from build123d import *

# Parameters (mm, degrees)
SKETCH1_W           = 52
SKETCH1_H           = 38
BULK_EXTRUDE_DEPTH  = 3
FILLET1_R           = 7
SKETCH2_R           = 31.5
MOTOR_SUPPORT_DEPTH = 3
SKETCH3_R           = 6
WIRE_PASSTHRU_DEPTH = 143.168954603
FILLET2_R           = 10


with BuildPart() as part:
    # Sketch1 → BULK EXTRUDE (new body)
    # profile 1 of 3: a face of its own
    with BuildSketch(Plane.ZY.offset(19)):
        with BuildLine():
            Line((-2, -62.201941274), (-2, -24.5))
            Line((-2, -24.5), (-2, 25.456486729))
            ThreePointArc((-2, 25.456486729), (-115, -18.372727273), (-2, -62.201941274))
        make_face()
        with Locations((-57, 0)):
            Rectangle(SKETCH1_W, SKETCH1_H, mode=Mode.SUBTRACT)
    # profile 2 of 3: a face of its own
    with BuildSketch(Plane.ZY.offset(19)):
        with Locations((-57, 0)):
            Rectangle(SKETCH1_W, SKETCH1_H)
    # profile 3 of 3: a face of its own
    with BuildSketch(Plane.ZY.offset(19)):
        with BuildLine():
            Line((14.71055964, -24.5), (-2, -24.5))
            Line((-2, -24.5), (-2, -62.201941274))
            ThreePointArc((-2, -62.201941274), (9.424545918, -44.711355605), (14.71055964, -24.5))
        make_face()
    extrude(amount=BULK_EXTRUDE_DEPTH)

    # Fillet1
    fillet1_edges = [part.edges().sort_by_distance(p)[0] for p in [
        (-20.5, -24.5, -2),
        (-20.5, -24.5, 14.71055964),
        (-20.5, 25.456486729, -2),
    ]]
    fillet(fillet1_edges, radius=FILLET1_R)

    # Sketch2 → MOTOR SUPPORT (add)
    with BuildSketch(Plane.ZY.offset(22)):
        with Locations(Location((-50, -18.372727273, 0), (0, 0, 270))):
            Circle(SKETCH2_R)
    extrude(amount=MOTOR_SUPPORT_DEPTH)

    # Sketch3 → WIRE PASSTHRU (cut, through all)
    with BuildSketch(Plane.ZY.offset(25)):
        with Locations(Location((-50, -18.372727273, 0), (0, 0, 270))):
            Circle(SKETCH3_R)
    extrude(amount=-WIRE_PASSTHRU_DEPTH, mode=Mode.SUBTRACT)

    # Fillet2
    # the kernel refuses this fillet: 10 mm, written as the material it takes off along each edge
    with BuildSketch(Plane(origin=(-19, -18.372727273, -50), x_dir=(0, -1, 0), z_dir=(0, 0, -1))) as fillet2_piece_1:
        with BuildLine():
            CenterArc((15.16515139, 10), FILLET2_R, 203.578178478, 66.421821522)
            Line((6, 6), (5.816696972, 5.92))
            ThreePointArc((5.816696972, 5.92), (5.8, 3), (5.8, 0))
            Line((5.8, 0), (6, -0.2))
            Line((6, -0.2), (15.16515139, -0.2))
            Line((15.16515139, -0.2), (15.16515139, 0))
        make_face()
    revolve(axis=Axis((-19, -18.372727273, -50), (-1, 0, 0)), mode=Mode.SUBTRACT)


solid = part.part
Work out the finished part from the listing and answer in its coordinate system (mm). A direction names the side the tool comes from. Coordinates: 2 decimals unless noted, no trailing zeros. Loops run counter-clockwise (first coordinate to the right, second up) from the corner with the lowest first, then second, coordinate; pieces in that order, holes last. Notation, with made-up numbers: M -0.75,85 L 4.25,85 A21 ccw 4.25,118 Z; hole C 58,22.5 d7. An arc over 180 degrees is marked long. Answer in a Markdown table with one row per item. Add a question column.
1. Find section A-A, the plane z = -50. Write down the section's boundary in (x, y).
2. Find section D-D, the plane y = 24.5. Write down the section's boundary in (x, z), then the cut area to 3 significant figures.
3. Find section B-B, the plane x = -23.5. Write down the section's boundary in (y, z).
4. Flat-ended cylindrical pins translate along their axes: P1, Ø1.5, axis at y = -46.5, z = -93, coming from the -X side; P2, Ø3.5, axis at x = -20.5, y = 4.5, coming from the +Z side; P3, Ø2, axis at x = -22, z = -7.5, coming from the -Y side. Find the tip coordinate at first contact, or state that the pin passes through.
5. Consider L1, parallel to Z at x = -24.25, y = -17; L2, parallel to X at y = 33, z = -49; L3, parallel to Z at x = -20.5, y = -22.5. Determine where each line is inside the solid, lowest interval first.
6. Find section C-C, the plane z = -26. Write down the section's boundary in (x, y).
7. A tool of negligible diameter and unlimited length cuts with its end or side. For faces 1 (the flat face through (-20, 2, -2)), 2 (the cylindrical face through (-23.479, -47.471, -62.065)), 3 (the flat face through (-25, -18, -57)), from which of +Z, -Z, +X, -X, +Y, -Y can it reach the whole face along a straight path? Write none if from no direction.
Reported:
| question | item | result |
|---|---|---|
| 1 | outline | M -25,-49.87 L -22,-49.87 L -22,-83.37 L -19,-83.37 L -19,-33.54 A10 ccw -25,-24.37 Z; M -25,-12.37 A10 ccw -19,-3.21 L -19,46.63 L -22,46.63 L -22,13.13 L -25,13.13 Z |
| 2 | outline | M -22,-98.86 L -19,-98.86 L -19,-2.25 L -22,-2.25 Z |
| 2 | area | 290 mm^2 |
| 3 | outline | C -18.37,-50 d63; hole C -18.37,-50 d13.63 |
| 4 | P1 | stops at x = -22 |
| 4 | P2 | stops at z = -2 |
| 4 | P3 | stops at y = -68.4 |
| 5 | L1 | z = -81.47 to -56.22, -43.78 to -18.53 |
| 5 | L2 | x = -22 to -19 |
| 5 | L3 | z = -114.87 to -59, -41 to 0.1 |
| 6 | outline | M -25,-38.77 L -22,-38.77 L -22,-78.78 L -19,-78.78 L -19,42.03 L -22,42.03 L -22,2.03 L -25,2.03 Z |
| 7 | face 1 | +Z, +X, -X, +Y |
| 7 | face 2 | -X |
| 7 | face 3 | +Z, -Z, -X, +Y, -Y |
